```python
from build123d import *

# Parameters (mm, degrees)
F0_W     = 34.4
F0_H     = 15.2
F0_R     = 1.935
F1_DEPTH = 51.2
F2_DEPTH = 1.5
F3_R     = 2
F4_R     = 0.75


with BuildPart() as f1:
    # F0 (on Front) → F1 (new body)
    with BuildSketch(Plane.XZ):
        with Locations((17.2, 7.6)):
            Rectangle(F0_W, F0_H)
        with Locations((13.795, 5.145)):
            Circle(F0_R, mode=Mode.SUBTRACT)
        with Locations((13.795, 5.145)):
            Circle(F0_R)
    extrude(amount=F1_DEPTH)

    # F0 (on Front) → F2 (join)
    with BuildSketch(Plane.XZ):
        with Locations((13.795, 5.145)):
            Circle(F0_R)
    extrude(amount=-F2_DEPTH)

    # F3
    f3_edges = [f1.edges().sort_by_distance(p)[0] for p in [
        (34.4, 0, 7.6),
        (0, 0, 7.6),
    ]]
    fillet(f3_edges, radius=F3_R)

    # F4
    f4_edges = [f1.edges().sort_by_distance(p)[0] for p in [
        (34.4, -26.6, 15.2),
    ]]
    fillet(f4_edges, radius=F4_R)


solid = f1.part
```
Here's how the part is built. I have some questions about the finished solid (model axes, mm). A direction names the side the tool comes from. Give positions to 0.01 mm unless a question says otherwise; leave off trailing zeros. Loops run counter-clockwise (first coordinate to the right, second up) from the corner with the lowest first, then second, coordinate; pieces in that order, holes last. Notation, with made-up numbers: M 39,89.25 L 66,89.25 A13 ccw 66,106.25 Z; hole C 75.25,15 d5. An arc over 180 degrees is marked long. Return JSON: item names as keys, results as strings.
Item 1: I'm going to push a flat-ended pin straight in: pin 1 Ø2 at (x, z) = (29.5, 6.5) entering from +Y. Where does the tip first touch, or does it pass through?
A:
{"pin 1": "stops at y = 0"}
Item 2: Imagine slicing it at B-B on x = 16.5. List the corners of the cut face in (y, z) for me, then the cut area to 3 significant figures.
A:
{"outline": "M -51.2,0 L 0,0 L 0,14.45 A0.75 ccw -0.75,15.2 L -51.2,15.2 Z", "area": "778 mm^2"}
Item 3: Please list where these lines run through material, in increasing order: line 1 (Y direction, x = 9, z = 13); line 2 (X direction, y = -1, z = 10.75); line 3 (X direction, y = -47.5, z = 14.75).
A:
{"line 1": "y = -51.2 to 0", "line 2": "x = 0.27 to 34.13", "line 3": "x = 0.06 to 34.34"}
Item 4: On a 3-axis mill with a long thin cutter (end or side, diameter ignored), from which of +Z, -Z, +X, -X, +Y, -Y can I reach the whole of each face in a straight line? I mean faces 1 (the flat face through (17, -25, 0)), 2 (the cylindrical face through (15.64, 0.74, 5.73)). Say none if no direction works.
A:
{"face 1": "-Z, +X, -X, +Y, -Y", "face 2": "+Y"}
Item 5: Imagine slicing it at A-A on z = 13. List the corners of the cut face in (x, y) for me, then the cut area to 3 significant figures.
A:
{"outline": "M 0,-51.2 L 34.4,-51.2 L 34.4,-2 A2 ccw 32.4,0 L 2,0 A2 ccw 0,-2 Z", "area": "1,760 mm^2"}
